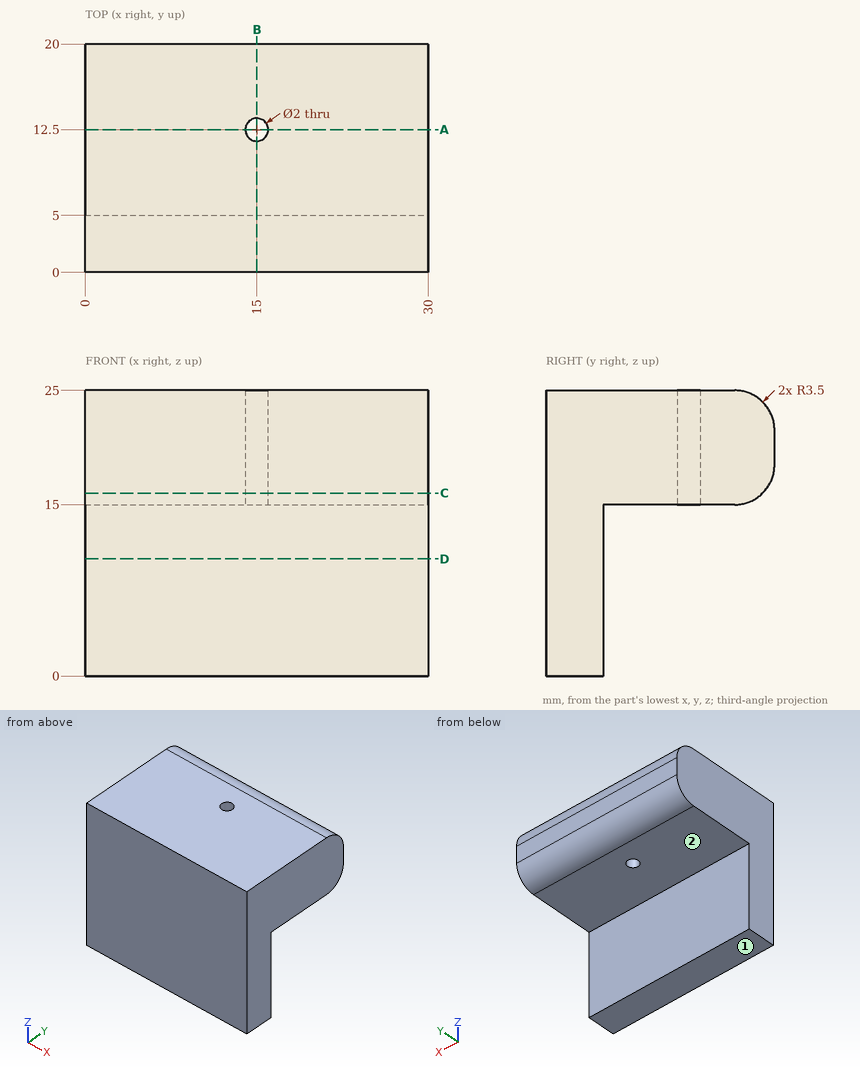
Geometry check sheet. Reference: drawing and pictorial views, mm from the part's lowest x, y, z. A direction names the side the tool comes from. Coordinates: 2 decimals unless noted, no trailing zeros. Loops run counter-clockwise (first coordinate to the right, second up) from the corner with the lowest first, then second, coordinate; pieces in that order, holes last.
1) Sectioned sample at D-D (z = 10.25). Record the boundary of the cut face in (x, y).
2) Sectioned sample at B-B (x = 15). Record the boundary of the cut face in (y, z), and give its area (3 significant figures).
3) Access from +Z, -Z, +X, -X, +Y, -Y to the whole of each face (thin tool, end or side, straight path). Record for the marked faces 1 and 2.
4) Gauge pin test, flat ends, axial feed: pin 1 (5 mm diameter, centred on x = 7.5, z = 14.5, fed in from +Y); pin 2 (1 mm diameter, centred on x = 23.5, y = 13.5, fed in from -Z); pin 3 (7.5 mm diameter, centred on x = 17, z = 11, fed in from +Y). Record the tip position at first contact, or that the pin passes through.
5) Material ranges on probe 1 along Y at (x, z) = (15, 20.5); probe 2 along Z at (x, y) = (14.5, 14.25); probe 3 along Y at (x, z) = (15, 22.25), recorded low to high.
6) Sectioned sample at A-A (y = 12.5). Record the boundary of the cut face in (x, z), and give its area (3 significant figures).
7) Sectioned sample at C-C (z = 16). Record the boundary of the cut face in (x, y), and give its area (3 significant figures).
Check sheet entries:
1. outline: (0, 0) - (30, 0) - (30, 5) - (0, 5) - close
2. outline: (0, 0) - (5, 0) - (5, 15) - (11.5, 15) - (11.5, 25) - (0, 25) - close; (13.5, 15) - (16.5, 15) arc R3.5 ccw to (20, 18.5) - (20, 21.5) arc R3.5 ccw to (16.5, 25) - (13.5, 25) - close
2. area: 250 mm2
3. face 1: -Z, +X, -X, +Y, -Y
3. face 2: -Z, +X, -X, +Y
4. pin 1: stops at y = 19.66
4. pin 2: stops at z = 15
4. pin 3: stops at y = 5
5. probe 1: y = 0 to 11.5, 13.5 to 20
5. probe 2: z = 15 to 25
5. probe 3: y = 0 to 11.5, 13.5 to 19.92
6. outline: (0, 15) - (14, 15) - (14, 25) - (0, 25) - close; (16, 15) - (30, 15) - (30, 25) - (16, 25) - close
6. area: 280 mm2
7. outline: (0, 0) - (30, 0) - (30, 18.95) - (0, 18.95) - close; hole circle Ø2 at (15, 12.5)
7. area: 565 mm2
